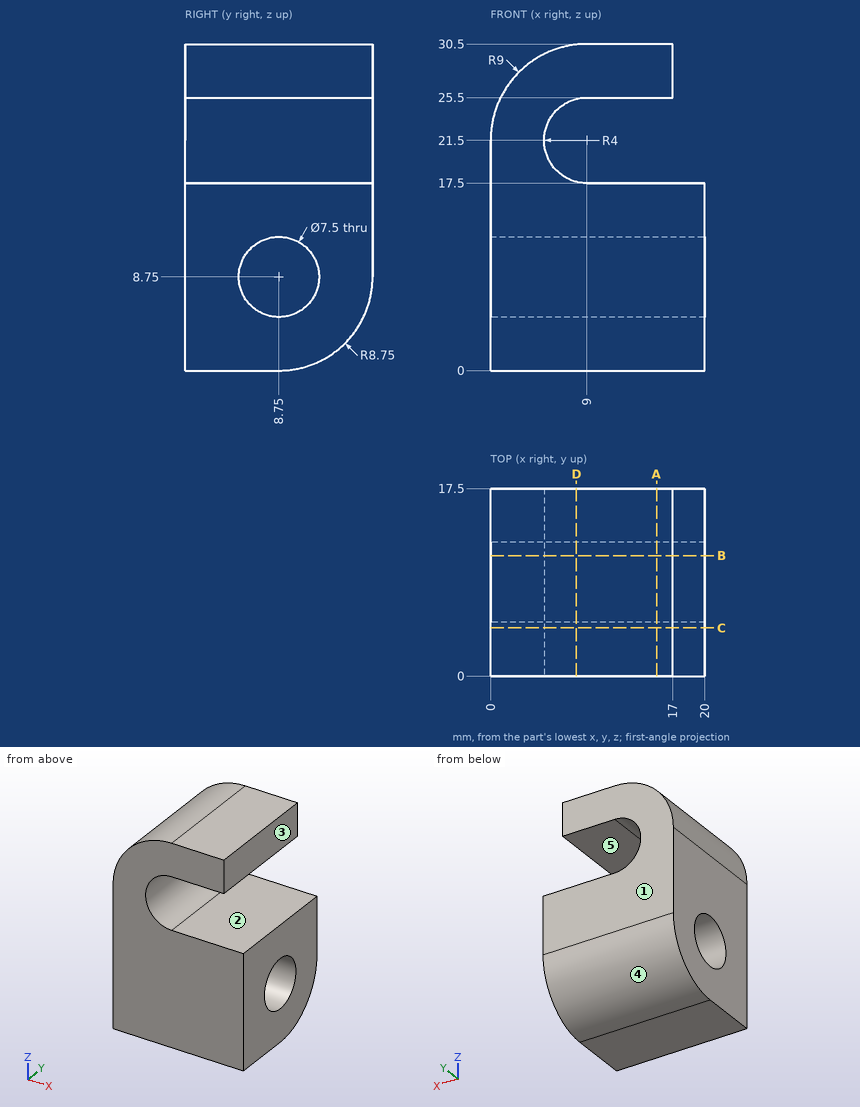
Check sheet for the drawn part. Datum: minimum x, y, z corner. Units: mm. A direction names the side the tool comes from. Give positions to 0.01 mm unless a question says otherwise; leave off trailing zeros. Order: outer loops, then holes, each group sorted by start corner. A loop starts at its lowest first (then second) coordinate and runs counter-clockwise, first axis right, second up. Notation, with made-up numbers: (47, -18.75) -> (101, -18.75) arc R19 cw to (101, -11.75) -> close; hole circle Ø3 at (48, -39). An arc over 180 degrees is marked (long way). Use a Markdown table: item, result.
1) Depth check by flat-ended pin: pin 1 Ø2 at (x, z) = (11, 15) entering from -Y; pin 2 Ø1.5 at (y, z) = (6.5, 23) entering from +X; pin 3 Ø2 at (y, z) = (3.5, 25.5) entering from +X; pin 4 Ø5 at (x, y) = (5.5, 15.5) entering from +Z. Enter the tip coordinate at first touch or a pass-through.
Results:
| item | result |
|---|---|
| pin 1 | y = 0 |
| pin 2 | x = 5.69 |
| pin 3 | x = 17 |
| pin 4 | z = 30.44 |
2) Section check D-D, the plane x = 8. Record the boundary of the cut face in (y, z).
Results:
| item | result |
|---|---|
| outline | (0, 0) -> (8.75, 0) arc R8.75 ccw to (17.5, 8.75) -> (17.5, 17.63) -> (0, 17.63) -> close; (0, 25.37) -> (17.5, 25.37) -> (17.5, 30.44) -> (0, 30.44) -> close; hole circle Ø7.5 at (8.75, 8.75) |
3) Section check A-A, the plane x = 15.5. Record the boundary of the cut face in (y, z).
Results:
| item | result |
|---|---|
| outline | (0, 0) -> (8.75, 0) arc R8.75 ccw to (17.5, 8.75) -> (17.5, 17.5) -> (0, 17.5) -> close; (0, 25.5) -> (17.5, 25.5) -> (17.5, 30.5) -> (0, 30.5) -> close; hole circle Ø7.5 at (8.75, 8.75) |
4) Mould release check, pull along Z, two halves, no side actions. Record for the marked faces 3, 4 and 5: pulls with the +Z half, pulls with the -Z half, needs draft (parallel to the pull), parting line crosses it, or undercut.
Results:
| item | result |
|---|---|
| face 3 | needs draft |
| face 4 | pulls with the -Z half |
| face 5 | undercut |
5) Material ranges on probe 1 along Z at (x, y) = (15.5, 5.75); probe 2 along Y at (x, z) = (6.75, 8.75); probe 3 along Z at (x, y) = (10, 1.25), recorded low to high.
Results:
| item | result |
|---|---|
| probe 1 | 0 to 6.5, 11 to 17.5, 25.5 to 30.5 |
| probe 2 | 0 to 5, 12.5 to 17.5 |
| probe 3 | 0 to 17.5, 25.5 to 30.5 |
6) Section check C-C, the plane y = 4.5. Record the boundary of the cut face in (x, z), then the cut area to 3 significant figures.
Results:
| item | result |
|---|---|
| outline | (0, 0) -> (20, 0) -> (20, 17.5) -> (9, 17.5) arc R4 cw to (9, 25.5) -> (17, 25.5) -> (17, 30.5) -> (9, 30.5) arc R9 ccw to (0, 21.5) -> close |
| area | 464 mm² |
7) Section check B-B, the plane y = 11.25. Record the boundary of the cut face in (x, z), then the cut area to 3 significant figures.
Results:
| item | result |
|---|---|
| outline | (0, 0.36) -> (20, 0.36) -> (20, 5.95) -> (0, 5.95) -> close; (0, 11.55) -> (20, 11.55) -> (20, 17.5) -> (9, 17.5) arc R4 cw to (9, 25.5) -> (17, 25.5) -> (17, 30.5) -> (9, 30.5) arc R9 ccw to (0, 21.5) -> close |
| area | 345 mm² |
8) Tool access check on the marked faces 1 and 2. Record the directions out of +Z, -Z, +X, -X, +Y, -Y that give a thin tool (end or side, any length) a straight path to the whole face; none if there is none.
Results:
| item | result |
|---|---|
| face 1 | +Z, -Z, +X, -X, +Y |
| face 2 | +X, +Y, -Y |
